Autodesk Inventor part; units mm, degrees
ref_plane "YZ Plane" through (0, 0, 0) normal (1, 0, 0) x (0, 1, 0)
ref_plane "XZ Plane" through (0, 0, 0) normal (0, 1, 0) x (-1, 0, 0)
ref_plane "XY Plane" through (0, 0, 0) normal (0, 0, 1) x (1, 0, 0)
sketch "Sketch1" plane through (0, 0, 0) normal (0, 1, 0) x (-1, 0, 0)
  circle A0 centre (0, 0) radius 14.25
  dimension "d0" = 28.5
extrude "Extrusion1" add sketch "Sketch1" along normal blind 5
sketch "Sketch2" plane through (0, 5, 0) normal (0, 1, 0) x (1, 0, 0)
  circle A0 centre (0, 0) radius 14.25
  circle A1 centre (0, 0) radius 7.9
  dimension "d3" = 15.8
extrude "Extrusion2" add sketch "Sketch2" along normal blind 20 contours A1
sketch "Sketch3" plane through (0, 25, 0) normal (0, 1, 0) x (1, 0, 0)
  circle A0 centre (0, 0) radius 7.9
  circle A1 centre (0, 0) radius 4
  dimension "d6" = 8
extrude "Extrusion3" cut sketch "Sketch3" against normal blind 25.6 contours A1
chamfer "Chamfer1" distance 0.5 angle 45 1 edges at (-7.9, 25, 0)
chamfer "Chamfer2" distance 0.5 angle 45 3 edges at (-7.9, 5, 0) (14.25, 5, 0) (14.25, 0, 0)
thread "Thread1"
sketch "Sketch5" plane through (0, 0, 0) normal (0, -1, 0) x (1, 0, 0)
  circle A0 centre (0, 0) radius 4
  circle A1 centre (0, 0) radius 13.75
  line L0 (0, 0) -> (-13.75, 0) construction
  line L1 (0, 0) -> (13.75, 0) construction
  circle A2 centre (0, 0) radius 13.75 construction
  line L2 (0, 0) -> (0, 13.75) construction
  line L3 (0, 0) -> (0, -13.75) construction
  circle A3 centre (0, 11) radius 1.5
  circle A4 centre (11, 0) radius 1.5
  circle A5 centre (-11, 0) radius 1.5
  circle A6 centre (0, -11) radius 1.5
  dimension "d28" = 11
  dimension "d29" = 3
  dimension "d30" = 11
  dimension "d31" = 11
  dimension "d32" = 11
extrude "Extrusion5" cut sketch "Sketch5" against normal up to surface (5 mm away) contours A3 | A4 | A5 | A6
properties part number "ZACMENut" material "ABS Plastic"
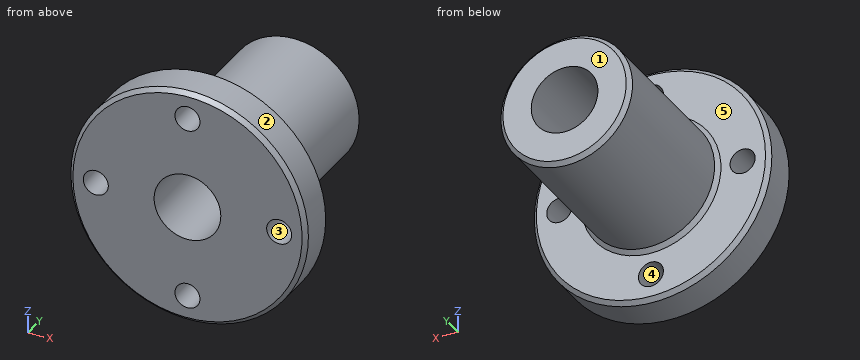
Design review of the part built by this model. Coordinates are the model's own, in mm. Face numbers are marked on the shaded views. A direction names the side the tool comes from. Round coordinates to 2 decimals unless told otherwise and drop trailing zeros. Order: outer loops, then holes, each group sorted by start corner. A loop starts at its lowest first (then second) coordinate and runs counter-clockwise, first axis right, second up. Notation, with made-up numbers: (54, 22) - (66, 22) arc R34 ccw to (66, 57) - close; hole circle Ø2 at (79.5, 12). An arc over 180 degrees is marked (long way). Return JSON: item names as keys, results as strings.
Q1. The part is to be moulded in two halves that separate along X. For the marked faces 1, 2 and 3, say which applies: pulls with the +X half, pulls with the -X half, needs draft (parallel to the pull), parting line crosses it, or undercut.
Computed values:
{"face 1": "needs draft", "face 2": "parting line crosses it", "face 3": "undercut"}
Q2. Consider section A-A on x = 0. Write out the cut boundary in (y, z), plus the area to 3 significant figures.
Computed values:
{"outline": "(0, -13.75) - (0.5, -14.25) - (4.5, -14.25) - (5, -13.75) - (5, -12.5) - (0, -12.5) - close; (0, -9.5) - (5, -9.5) - (5, -8.4) - (5.5, -7.9) - (24.5, -7.9) - (25, -7.4) - (25, -4) - (0, -4) - close; (0, 4) - (25, 4) - (25, 7.4) - (24.5, 7.9) - (5.5, 7.9) - (5, 8.4) - (5, 9.5) - (0, 9.5) - close; (0, 12.5) - (5, 12.5) - (5, 13.75) - (4.5, 14.25) - (0.5, 14.25) - (0, 13.75) - close", "area": "228 mm2"}
Q3. For pin 1 Ø10 at (y, z) = (18.5, 9) entering from +X; pin 2 Ø10 at (x, y) = (8, 16.5) entering from -Z; pin 3 Ø4 at (x, z) = (-10, 6.5) entering from +Y, all flat-tipped, find the tip position at first contact; note any pin that passes through.
Computed values:
{"pin 1": "stops at x = 6.81", "pin 2": "stops at z = -7.31", "pin 3": "stops at y = 5"}
Q4. Machinability: for the marked faces 4 and 5, which of the approach directions +Z, -Z, +X, -X, +Y, -Y give a long, thin tool a straight path to every point of the face, cutting with its end or side? Answer none if there is none.
Computed values:
{"face 4": "+Y, -Y", "face 5": "+Y"}
Q5. Consider section B-B on y = 22.5. Write out the cut boundary in (x, z).
Computed values:
{"outline": "circle Ø15.8 at (0, 0); hole circle Ø8 at (0, 0)"}
Q6. Wall thickness on L1, parallel to Z at x = 0, y = 3.5; L2, parallel to X at y = 19.75, z = -0.25; L3, parallel to Y at x = -12.75, z = 0.75: over which ranges is each line inside the solid? List them lowest first. Write a range as [from, to].
Computed values:
{"L1": "z = [-14.25, -12.5], [-9.5, -4], [4, 9.5], [12.5, 14.25]", "L2": "x = [-7.9, -3.99], [3.99, 7.9]", "L3": "y = [0, 5]"}
Q7. Consider section C-C on z = -1. Give the number of separate pieces and of enclosed holes in the cut face, plus the area to 3 significant figures.
Computed values:
{"separate pieces": "4", "enclosed holes": "0", "area": "239 mm2"}
